Autodesk Inventor part; units mm, degrees
ref_plane "YZ Plane" through (0, 0, 0) normal (1, 0, 0) x (0, 1, 0)
ref_plane "XZ Plane" through (0, 0, 0) normal (0, 1, 0) x (-1, 0, 0)
ref_plane "XY Plane" through (0, 0, 0) normal (0, 0, 1) x (1, 0, 0)
sketch "Sketch1" plane through (0, 0, 0) normal (0, 0, 1) x (1, 0, 0)
  circle A0 centre (0, 0) radius 18.5
  dimension "d0" = 37
extrude "Extrusion1" add sketch "Sketch1" against normal blind 22
sketch "Sketch2" plane through (0, 0, -22) normal (0, 0, -1) x (-1, 0, 0)
  circle A0 centre (0, 0) radius 18.5
  circle A1 centre (0, 0) radius 16.5
  dimension "d3" = 33
extrude "Extrusion2" add sketch "Sketch2" along normal blind 25 contours A1
sketch "Sketch3" plane through (0, 0, -47) normal (0, 0, -1) x (-1, 0, 0)
  circle A0 centre (0, 0) radius 18.5
  circle A1 centre (0, 0) radius 7
  dimension "d6" = 14
extrude "Extrusion3" add sketch "Sketch3" along normal blind 6.5 contours A1
sketch "Sketch4" plane through (0, 0, -53.5) normal (0, 0, -1) x (-1, 0, 0)
  circle A0 centre (0, 0) radius 1
  dimension "d9" = 2
extrude "Extrusion4" add sketch "Sketch4" along normal blind 1.5
sketch "Sketch5" plane through (0, 0, -47) normal (0, 0, -1) x (-1, 0, 0)
  line L0 (-20.5, -8.75) -> (-13.5, -8.75)
  line L1 (-13.5, -8.75) -> (-13.5, 8.75)
  line L2 (-13.5, 8.75) -> (-20.5, 8.75)
  line L3 (-20.5, 8.75) -> (-20.5, -8.75)
  circle A0 centre (0, 0) radius 16.5
  dimension "d12" = 17.5
  dimension "d13" = 7
  dimension "d14" = 8.75
  dimension "d15" = 37
extrude "Extrusion5" add sketch "Sketch5" along normal blind 5.8 contours L3 L2 A0 L0 | A0 L2 L1 L0 picked at (-14.4657, -0.6136)
sketch "Sketch6" plane through (20.5, -8.75, -47) normal (1, 0, 0) x (0, 0, -1)
  line L0 (5.3, 17) -> (0.5, 17)
  line L1 (0.5, 17) -> (0.5, 0.5)
  line L2 (0.5, 0.5) -> (5.3, 0.5)
  line L3 (5.3, 0.5) -> (5.3, 17)
  line L4 (0, 17.5) -> (5.8, 17.5)
  line L5 (5.8, 17.5) -> (5.8, 0)
  line L6 (0, 0) -> (5.8, 0)
  line L7 (0, 17.5) -> (0, 0)
  line L8 (3.8, 15.25) -> (3.3, 15.25)
  line L9 (3.3, 15.25) -> (3.3, 14.75)
  line L10 (3.3, 14.75) -> (3.8, 14.75)
  line L11 (3.8, 14.75) -> (3.8, 15.25)
  line L12 (3.8, 12.75) -> (3.3, 12.75)
  line L13 (3.8, 12.25) -> (3.8, 12.75)
  line L14 (3.3, 12.25) -> (3.8, 12.25)
  line L15 (3.3, 12.75) -> (3.3, 12.25)
  line L16 (3.8, 10.25) -> (3.3, 10.25)
  line L17 (3.8, 9.75) -> (3.8, 10.25)
  line L18 (3.3, 9.75) -> (3.8, 9.75)
  line L19 (3.3, 10.25) -> (3.3, 9.75)
  line L20 (3.8, 7.75) -> (3.3, 7.75)
  line L21 (3.8, 7.25) -> (3.8, 7.75)
  line L22 (3.3, 7.25) -> (3.8, 7.25)
  line L23 (3.3, 7.75) -> (3.3, 7.25)
  line L24 (3.8, 5.25) -> (3.3, 5.25)
  line L25 (3.8, 4.75) -> (3.8, 5.25)
  line L26 (3.3, 4.75) -> (3.8, 4.75)
  line L27 (3.3, 5.25) -> (3.3, 4.75)
  line L28 (3.8, 2.75) -> (3.3, 2.75)
  line L29 (3.8, 2.25) -> (3.8, 2.75)
  line L30 (3.3, 2.25) -> (3.8, 2.25)
  line L31 (3.3, 2.75) -> (3.3, 2.25)
  line L32 (0, 17.5) -> (5.8, 17.5)
  line L33 (4.3185, 17) -> (3.8, 17)
  line L34 (3.8, 17) -> (3.8, 17.5)
  line L35 (3.8, 17.5) -> (4.3185, 17.5)
  line L36 (4.3185, 17.5) -> (4.3185, 17)
  line L37 (3.8, 0.5) -> (4.3185, 0.5)
  line L38 (4.3185, 0.5) -> (4.3185, 0)
  line L39 (4.3185, 0) -> (3.8, 0)
  line L40 (3.8, 0) -> (3.8, 0.5)
  line L41 (5.8, 15.25) -> (5.3, 15.25)
  line L42 (5.3, 15.25) -> (5.3, 14.75)
  line L43 (5.3, 14.75) -> (5.8, 14.75)
  line L44 (5.8, 14.75) -> (5.8, 15.25)
  line L45 (5.8, 2.75) -> (5.3, 2.75)
  line L46 (5.3, 2.75) -> (5.3, 2.25)
  line L47 (5.3, 2.25) -> (5.8, 2.25)
  line L48 (5.8, 2.25) -> (5.8, 2.75)
  point P0 (-47, 8.75)
  dimension "d18" = 0.5
  dimension "d19" = 0.5
  dimension "d20" = 0.5
  dimension "d21" = 0.5
  dimension "d22" = 0.5
  dimension "d23" = 0.5
  dimension "d26" = 2.5
  dimension "d31" = 1.5
  dimension "d32" = 1.75
extrude "Extrusion6" cut sketch "Sketch6" against normal blind 5.5 contours L3 L2 L1 L0
extrude "Extrusion7" cut sketch "Sketch6" against normal blind 3.6 contours L0 L34 L4 L36 | L41 L5 L43 L3 | L45 L5 L47 L3 | L2 L38 L6 L40
sketch "Sketch7" plane through (0, 0, 0) normal (0, 0, 1) x (1, 0, 0)
  circle A0 centre (-8, 14) radius 1.25
  circle A1 centre (-16, 0) radius 1.5
  circle A2 centre (-8, -14) radius 1.25
  circle A3 centre (8, -14) radius 1.25
  circle A4 centre (16, 0) radius 1.5
  circle A5 centre (8, 14) radius 1.25
  circle A6 centre (0, -7) radius 6
  point P0 (0, 0)
  dimension "d37" = 12
  dimension "d38" = 7
extrude "Extrusion8" add sketch "Sketch7" along normal blind 5.8 contours A6
sketch "Sketch8" plane through (0, -7, 5.8) normal (0, 0, 1) x (1, 0, 0)
  circle A0 centre (0, 7) radius 7
  circle A1 centre (0, 0) radius 3
  dimension "d41" = 6
extrude "Extrusion9" add sketch "Sketch8" along normal blind 14 contours A1 A0 | A0 A1 picked at (-0.8611, 0.9867) picked at (-1.0544, -0.7781)
sketch "Sketch9" plane through (0, -7, 19.8) normal (0, 0, 1) x (1, 0, 0)
  line L0 (2.4, 2.1786) -> (4.1019, 2.1786)
  line L1 (4.1019, 2.1786) -> (4.1019, -2.6301)
  line L2 (4.1019, -2.6301) -> (2.4, -2.6301)
  line L3 (2.4, -2.6301) -> (2.4, 2.1786)
  circle A0 centre (0, 0) radius 3
  point P0 (0, 7)
  dimension "d44" = 5.4
extrude "Extrusion10" cut sketch "Sketch9" against normal blind 11 contours L0 L1 L2 L3 A0 | A0 L3 picked at (2.5094, 0.416)
extrude "Extrusion11" cut sketch "Sketch7" against normal blind 10 contours A0 | A1 | A2 | A3 | A4 | A5
properties part number "Motor"
Part model, mm, in its own coordinate system. A direction names the side the tool comes from. Coordinates: 2 decimals unless noted, no trailing zeros. Loops run counter-clockwise (first coordinate to the right, second up) from the corner with the lowest first, then second, coordinate; pieces in that order, holes last. Notation, with made-up numbers: M -6.5,74 L 13.5,74 A21 cw 13.5,80 Z; hole C 77.5,64.25 d3. An arc over 180 degrees is marked long. Use a Markdown table: item, result. Add a question column.
Q1. Cut at B-B (x = -8). Write the cut outline in (y, z).
Q2. Mould opens along X. For faces 1 (the flat face through (20.5, 0, -47.2)), 2 (the flat face through (-16, 0, -10)), 3 (the flat face through (18, 0, -47.5)), 4 (the flat face through (-8, -14, -10)) say: +X half, -X half, draft (parallel to the pull), parting line (faces both ways), or undercut.
Q3. Which spindle directions (+Z, -Z, +X, -X, +Y, -Y) get a long thin tool onto all of the face, cutting with end or side? Do faces 5 (the flat face through (2.4, -7, 14)), 6 (the cylindrical face through (-17.5, 0.07, -4.93)), 7 (the flat face through (18, 0, -52.3)), 8 (the flat face through (0, -7, 19.8)), 9 (the flat face through (-17, 0, -22)). Say none if no direction does.
Q4. Cut at A-A (z = -3). Write the cut outline in (x, y), and give its area (3 significant figures).
Q5. Pin check, flat tips, straight feed: P1, Ø6, axis at x = 12.5, y = 11.5, coming from the -Z side; P2, Ø1.2, axis at x = -8.5, y = -14.5, coming from the +Z side; P3, Ø2, axis at x = 4, y = 5, coming from the -Z side. Stop position of each tip, or through.
Q6. Cut at D-D (z = -12). Write the cut outline in (x, y).
Q7. Probe L1, parallel to Y at x = -8, z = -6; L2, parallel to Z at x = -5.5, y = -13; L3, parallel to Z at x = -5, y = 0. List the from-to ranges inside material, lowest first.
Worked out:
| question | item | result |
|---|---|---|
| 1 | outline | M -16.68,-22 L -14.43,-22 L -14.43,-47 L 14.43,-47 L 14.43,-22 L 16.68,-22 L 16.68,0 L 15.25,0 L 15.25,-10 L 12.75,-10 L 12.75,0 L -12.75,0 L -12.75,-10 L -15.25,-10 L -15.25,0 L -16.68,0 Z |
| 2 | face 1 | +X half |
| 2 | face 2 | undercut |
| 2 | face 3 | draft |
| 2 | face 4 | undercut |
| 3 | face 5 | +Z, +X, +Y, -Y |
| 3 | face 6 | +Z |
| 3 | face 7 | +X |
| 3 | face 8 | +Z, +X, -X, +Y, -Y |
| 3 | face 9 | none |
| 4 | outline | C 0,0 d37; hole C -16,0 d3; hole C -8,-14 d2.5; hole C -8,14 d2.5; hole C 8,-14 d2.5; hole C 8,14 d2.5; hole C 16,0 d3 |
| 4 | area | 1,040 mm2 |
| 5 | P1 | stops at z = -52.8 |
| 5 | P2 | stops at z = 0 |
| 5 | P3 | stops at z = -53.5 |
| 6 | outline | C 0,0 d37 |
| 7 | L1 | y = -16.68 to -15.25, -12.75 to 12.75, 15.25 to 16.68 |
| 7 | L2 | z = -47 to 0 |
| 7 | L3 | z = -53.5 to 0 |
